Work out the finished part from the listing and answer in its coordinate system (mm). Give positions to 0.01 mm unless a question says otherwise; leave off trailing zeros. Loops run counter-clockwise (first coordinate to the right, second up) from the corner with the lowest first, then second, coordinate; pieces in that order, holes last. Notation, with made-up numbers: (41.5, 87.5) - (62.5, 87.5) arc R33 ccw to (62.5, 116.5) - close; hole circle Ø8 at (7.5, -36). An arc over 180 degrees is marked (long way). One line per item, written item: value.
from build123d import *

# Parameters (mm, degrees)
SKETCH1_W             = 38.1
SKETCH1_H             = 19.05
SKETCH1_R             = 2.54
BOSS_EXTRUDE1_DEPTH   = 3.175
SKETCH2_R             = 1.5875
CUT_EXTRUDE1_DEPTH    = 4.175
F_2_5MM_DOWEL_HOLE1_D = 2.5
FILLET1_R             = 2.54


with BuildPart() as part:
    # Sketch1 → Boss-Extrude1 (new body)
    with BuildSketch(Plane(origin=(0, 0, 0), x_dir=(1, 0, 0), z_dir=(0, 1, 0))):
        Rectangle(SKETCH1_W, SKETCH1_H)
        Circle(SKETCH1_R, mode=Mode.SUBTRACT)
    extrude(amount=BOSS_EXTRUDE1_DEPTH)

    # Sketch2 → Cut-Extrude1 (cut, through all)
    with BuildSketch(Plane(origin=(0, 3.175, 0), x_dir=(1, 0, 0), z_dir=(0, 1, 0))):
        with Locations((-4.318, 4.318)):
            Circle(SKETCH2_R)
        with Locations((4.318, 4.318)):
            Circle(SKETCH2_R)
        with Locations((-4.318, -4.318)):
            Circle(SKETCH2_R)
        with Locations((4.318, -4.318)):
            Circle(SKETCH2_R)
    extrude(amount=-CUT_EXTRUDE1_DEPTH, mode=Mode.SUBTRACT)

    # Ø2.5mm Dowel Hole1 (through all)
    with Locations(Plane(origin=(0, 3.175, 0), x_dir=(1, 0, 0), z_dir=(0, 1, 0))):
        with Locations((12.7, 0), (-12.7, 0)):
            Hole(F_2_5MM_DOWEL_HOLE1_D / 2)

    # Fillet1
    fillet1_edges = [part.edges().sort_by_distance(p)[0] for p in [
        (19.05, 1.5875, 9.525),
        (-19.05, 1.5875, 9.525),
        (-19.05, 1.5875, -9.525),
        (19.05, 1.5875, -9.525),
    ]]
    fillet(fillet1_edges, radius=FILLET1_R)


solid = part.part
1. A flat-ended cylindrical pin translates along its axis: pin 1 Ø2 at (x, z) = (-12.7, 0) entering from +Y. Find the tip coordinate at first contact, or state that the pin passes through.
Output:
pin 1: passes through
2. Section C-C (z = -3.75) is taken. Write down the section's boundary in (x, y) (3 decimals), and give its area (3 significant figures).
Output:
outline: (-19.05, 0) - (-5.8, 0) - (-5.8, 3.175) - (-19.05, 3.175) - close; (-2.836, 0) - (2.836, 0) - (2.836, 3.175) - (-2.836, 3.175) - close; (5.8, 0) - (19.05, 0) - (19.05, 3.175) - (5.8, 3.175) - close
area: 102 mm²
3. Section B-B (x = -12.7) is taken. Write down the section's boundary in (y, z) (3 decimals).
Output:
outline: (0, -9.525) - (3.175, -9.525) - (3.175, -1.25) - (0, -1.25) - close; (0, 1.25) - (3.175, 1.25) - (3.175, 9.525) - (0, 9.525) - close
4. The mould has two halves that part along X. Classify faces 1 (the cylindrical face through (-13.855, 1.565, 0.479)), 2 (the flat face through (19.05, 2, 0)), 3 (the flat face through (0, 2, -9.525)): released by +X, released by -X, zero draft, split by the parting line, or undercut.
Output:
face 1: undercut
face 2: released by +X
face 3: zero draft
5. Find the intervals of material crossed by line 1 along X through (y, z) = (3.05, 4.25); line 2 along X through (y, z) = (0.3, 5); line 3 along X through (y, z) = (1.55, -0.5), in increasing order.
Output:
line 1: x = -19.05 to -5.9, -2.73 to 2.73, 5.9 to 19.05
line 2: x = -19.05 to -5.75, -2.88 to 2.88, 5.75 to 19.05
line 3: x = -19.05 to -13.85, -11.55 to -2.49, 2.49 to 11.55, 13.85 to 19.05
6. Section D-D (y = 2.05) is taken. Count the separate pieces of the cut face and the enclosed holes in it, and give its area (3 significant figures).
Output:
separate pieces: 1
enclosed holes: 7
area: 659 mm²
7. Section A-A (z = 0) is taken. Write down the section's boundary in (x, y) (3 decimals), and give its area (3 significant figures).
Output:
outline: (-19.05, 0) - (-13.95, 0) - (-13.95, 3.175) - (-19.05, 3.175) - close; (-11.45, 0) - (-2.54, 0) - (-2.54, 3.175) - (-11.45, 3.175) - close; (2.54, 0) - (11.45, 0) - (11.45, 3.175) - (2.54, 3.175) - close; (13.95, 0) - (19.05, 0) - (19.05, 3.175) - (13.95, 3.175) - close
area: 89.0 mm²
